Here's how the part is built. I have some questions about the finished solid (model axes, mm). Give positions to 0.01 mm unless a question says otherwise; leave off trailing zeros. Loops run counter-clockwise (first coordinate to the right, second up) from the corner with the lowest first, then second, coordinate; pieces in that order, holes last.
Q1. If we section it at A-A (z = -18): Please give me the cut outline in (x, y), plus the area to 3 significant figures.
Q2. If we section it at B-B (x = 0): Please give me the cut outline in (y, z).
Q3. If we section it at D-D (x = -17.5): Please give me the cut outline in (y, z).
Q4. I need wall thicknesses on line 1 (Z direction, x = -7.5, y = -0.45); line 2 (X direction, y = 0.85, z = -16); line 3 (Z direction, x = 0, y = 0.75). Which ranges of each line are inside material? Lowest first, please.
Q5. If we section it at C-C (y = -0.65): Please give me the cut outline in (x, z), plus the area to 3 significant figures.
Q6. Will this pin go through, and if not, where does the flat tip stop? P1, Ø1.5, axis at x = -2, y = 1, coming from the +Z side.
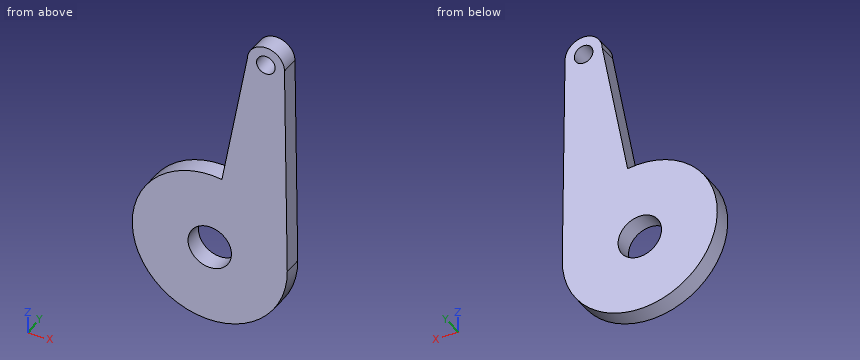
Autodesk Inventor part; units mm, degrees
ref_plane "YZ Plane" through (0, 0, 0) normal (1, 0, 0) x (0, 1, 0)
ref_plane "XZ Plane" through (0, 0, 0) normal (0, 1, 0) x (-1, 0, 0)
ref_plane "XY Plane" through (0, 0, 0) normal (0, 0, 1) x (1, 0, 0)
sketch "Boceto1" plane through (0, 0, 0) normal (0, 1, 0) x (-1, 0, 0)
  line L0 (0, -17.2515) -> (0, 17.2515) construction
  line L1 (-2.9997, 17.2904) -> (-3.4466, -17.089)
  arc A0 (2.999, 17.3273) -> (-2.9997, 17.2904) centre (0, 17.2515) ccw
  circle A1 centre (0, 17.2515) radius 1.5
  arc A2 (-3.4466, -17.089) -> (7.0947, -4.9057) centre (9.0523, -17.2515) ccw
  line L2 (0, -17.2515) -> (12.8049, -17.2515) construction
  line L3 (2.999, 17.3273) -> (7.0947, -4.9057)
  circle A3 centre (9.0523, -17.2515) radius 3.5
  point P0 (0, 0)
  point P1 (9.3192, -29.7486)
  point P2 (-0.0184, 20.2514)
  dimension "d0" = 6
  dimension "d1" = 3
  dimension "d3" = 12.5
  dimension "d4" = 50
  dimension "d5" = 7
extrude "Extrusión1" add sketch "Boceto1" along normal mid plane 3
equation "\"Radio_pliegue\" = Grosor"
equation "\"Anchura_desahogo_plegado\" = Grosor"
equation "\"Profundidad_desahogo_plegado\" = 0.5 * Grosor"
equation "\"Tamaño_destalonado\" = 4 * Grosor"
equation "\"Remanente_mínimo\" = 2 * Grosor"
equation "\"Radiodetransición\" = Radio_pliegue"
equation "\"Tamaño_de_radio_de_Jacobi\" = Radio_pliegue"
equation "\"TamañoSeparación\" = Grosor"
properties part number "Pinza_pieza4"
Check sheet entries:
1. outline: (-21.53, -1.5) - (-12.47, -1.5) - (-12.47, 1.5) - (-21.53, 1.5) - close; (-5.63, -1.5) - (3.43, -1.5) - (3.43, 1.5) - (-5.63, 1.5) - close
1. area: 54.4 mm2
2. outline: (-1.5, -25.87) - (1.5, -25.87) - (1.5, 15.75) - (-1.5, 15.75) - close; (-1.5, 18.75) - (1.5, 18.75) - (1.5, 20.25) - (-1.5, 20.25) - close
3. outline: (-1.5, -26.46) - (1.5, -26.46) - (1.5, -8.04) - (-1.5, -8.04) - close
4. line 1: z = -29.65 to -20.39, -14.11 to -4.85
4. line 2: x = -21.49 to -12.32, -5.78 to 3.43
4. line 3: z = -25.87 to 15.75, 18.75 to 20.25
5. outline: (-7.09, -4.91) arc R12.5 ccw (long way) to (3.45, -17.09) - (3, 17.29) arc R3 ccw to (-3, 17.33) - close; hole circle Ø7 at (-9.05, -17.25); hole circle Ø3 at (0, 17.25)
5. area: 672 mm2
6. P1: stops at z = 19.98
